Work out the finished part from the listing and answer in its coordinate system (mm). A direction names the side the tool comes from. Coordinates: 2 decimals unless noted, no trailing zeros. Order: outer loops, then holes, each group sorted by start corner. A loop starts at its lowest first (then second) coordinate and runs counter-clockwise, first axis right, second up. Notation, with made-up numbers: (-26.75, -24) - (26.25, -24) arc R12 cw to (26.25, -20) - close; hole circle Ø10 at (10, 44). An arc over 180 degrees is marked (long way). Answer as a JSON object with one key per item and string values. Group by question number.
1) The mould has two halves that part along X. Classify faces 3 (the face through (-72, 134.8, 18)), 4 (the face through (-59, 69, 38)), 5 (the face through (0, 67, 19)), 6 (the face through (-121.934, 49.426, 18.142)): released by +X, released by -X, zero draft, split by the parting line, or undercut.
2) Section C-C (y = 98) is taken. Give the vertices of the cut face in (x, z).
3) Each of these flat-tipped pins is pushed along its axis until it touches: P1, Ø18.5, axis at y = 67, z = 12.5, coming from the -X side; P2, Ø1, axis at y = 24, z = 17, coming from the -X side; P3, Ø3, axis at x = -30.5, z = 23.5, coming from the -Y side; P4, Ø1, axis at y = 33, z = 33.5, coming from the -X side. Where does it stop, or does it pass through?
4) Section A-A (z = 34.5) is taken. Give the vertices of the cut face in (x, y).
5) A tool of negligible diameter and unlimited length cuts with its end or side. For faces 1 (the face through (-150, 114, 19)), 2 (the face through (-147.657, 133.716, 18.142)), from which of +Z, -Z, +X, -X, +Y, -Y can it reach the whole face along a straight path? Write none if from no direction.
6) Section B-B (x = -85.5) is taken. Give the vertices of the cut face in (y, z), plus the area to 3 significant figures.
7) Find the intervals of material crossed by line 1 along X through (y, z) = (114, 19); line 2 along Y through (x, z) = (-25, 29); line 3 along Z through (x, y) = (-107, 69), in increasing order.
from build123d import *

# Parameters (mm, degrees)
EXTRUDE_1_DEPTH          = 38
SHELL_1_T                = -1.2
CUT_EXTRUDE_1_DEPTH      = 207.009708509
CUT_EXTRUDE_1_DEPTH_BACK = 207.009708509


with BuildPart() as part:
    # 草图1 → 凸台-拉伸1 (new body)
    with BuildSketch(Plane.XY):
        with BuildLine():
            Line((-150, 96), (-95, 0))
            Line((-95, 0), (0, 0))
            Line((0, 0), (0, 136))
            Line((0, 136), (-145, 136))
            ThreePointArc((-145, 136), (-148.535533906, 134.535533906), (-150, 131))
            Line((-150, 131), (-150, 96))
        make_face()
    extrude(amount=EXTRUDE_1_DEPTH)

    # 抽壳1
    shell_1_openings = [part.faces().sort_by_distance(p)[0] for p in [
        (-66.551705403, 73.332757841, 0),
    ]]
    offset(amount=SHELL_1_T, openings=shell_1_openings, kind=Kind.INTERSECTION)

    # 草图3 → 切除-拉伸1 (cut, two sides: drawn at the far end of the back side and taken through both)
    with BuildSketch(Plane.XZ.offset(-CUT_EXTRUDE_1_DEPTH_BACK)):
        with BuildLine():
            Line((-66, 7.25), (-74, 7.25))
            ThreePointArc((-74, 7.25), (-76.25, 5), (-74, 2.75))
            Line((-74, 2.75), (-66, 2.75))
            ThreePointArc((-66, 2.75), (-63.75, 5), (-66, 7.25))
        make_face()
        with BuildLine():
            Line((-26, 7.25), (-34, 7.25))
            ThreePointArc((-34, 7.25), (-36.25, 5), (-34, 2.75))
            Line((-34, 2.75), (-26, 2.75))
            ThreePointArc((-26, 2.75), (-23.75, 5), (-26, 7.25))
        make_face()
    extrude(amount=CUT_EXTRUDE_1_DEPTH + CUT_EXTRUDE_1_DEPTH_BACK, mode=Mode.SUBTRACT)


solid = part.part
Report:
{
 "1": {"face 3": "undercut", "face 4": "zero draft", "face 5": "released by +X", "face 6": "undercut"},
 "2": {"outline": "(-150, 0) - (-148.8, 0) - (-148.8, 36.8) - (-1.2, 36.8) - (-1.2, 0) - (0, 0) - (0, 38) - (-150, 38) - close"},
 "3": {"P1": "stops at x = -138.68", "P2": "stops at x = -109.04", "P3": "stops at y = 0", "P4": "stops at x = -114.19"},
 "4": {"outline": "(-150, 96) - (-95, 0) - (0, 0) - (0, 136) - (-145, 136) arc R5 ccw to (-150, 131) - close; hole (-148.8, 96.32) - (-94.3, 1.2) - (-1.2, 1.2) - (-1.2, 134.8) - (-145, 134.8) arc R3.8 ccw to (-148.8, 131) - close"},
 "5": {"face 1": "+Z, -Z, -X, +Y, -Y", "face 2": "-Z"},
 "6": {"outline": "(0, 0) - (1.2, 0) - (1.2, 36.8) - (134.8, 36.8) - (134.8, 0) - (136, 0) - (136, 38) - (0, 38) - close", "area": "252 mm²"},
 "7": {"line 1": "x = -150 to -148.8, -1.2 to 0", "line 2": "y = 0 to 1.2, 134.8 to 136", "line 3": "z = 36.8 to 38"}
}
